from build123d import *

# Parameters (mm, degrees)
SKETCH1_W           = 40
SKETCH1_H           = 8
SKETCH1_W_2         = 4
BOSS_EXTRUDE1_DEPTH = 7.5
BOSS_EXTRUDE2_START = 2.75
SKETCH1_5_W         = 40
SKETCH1_5_H         = 8
SKETCH1_5_H_2       = 2
SKETCH1_5_W_2       = 4
BOSS_EXTRUDE2_DEPTH = 4.75
SKETCH1_7_R         = 1.65
BOSS_EXTRUDE3_DEPTH = 2.3
CUT_EXTRUDE3_START  = 2.3
SKETCH3_R           = 4.5
CUT_EXTRUDE3_DEPTH  = 47.651506616


with BuildPart() as part:
    # Sketch1 → Boss-Extrude1 (new body)
    with BuildSketch(Plane(origin=(0, 0, 0), x_dir=(0, 0, -1), z_dir=(1, 0, 0))):
        with Locations((20, 0)):
            Rectangle(SKETCH1_W, SKETCH1_H)
        with Locations((38, 0)):
            Rectangle(SKETCH1_W_2, SKETCH1_H)
    extrude(amount=BOSS_EXTRUDE1_DEPTH)

    # Sketch1<5> → Boss-Extrude2 (add)
    with BuildSketch(Plane(origin=(0, 0, 0), x_dir=(0, 0, -1), z_dir=(1, 0, 0)).offset(BOSS_EXTRUDE2_START)):
        with Locations((20, 0)):
            Rectangle(SKETCH1_5_W, SKETCH1_5_H)
        with Locations((20, 5)):
            Rectangle(SKETCH1_5_W, SKETCH1_5_H_2)
        with Locations((38, 0)):
            Rectangle(SKETCH1_5_W_2, SKETCH1_5_H)
        with Locations((38, 5)):
            Rectangle(SKETCH1_5_W_2, SKETCH1_5_H_2)
    extrude(amount=BOSS_EXTRUDE2_DEPTH)

    # Sketch1<7> → Boss-Extrude3 (add)
    with BuildSketch(Plane(origin=(0, 0, 0), x_dir=(0, 0, -1), z_dir=(1, 0, 0))):
        with BuildLine():
            Line((44, 4), (40, 4))
            Line((40, 4), (40, -4))
            Line((40, -4), (44, -4))
            ThreePointArc((44, -4), (48, 0), (44, 4))
        make_face()
        with Locations((44, 0)):
            Circle(SKETCH1_7_R, mode=Mode.SUBTRACT)
    extrude(amount=BOSS_EXTRUDE3_DEPTH)

    # Sketch3 → Cut-Extrude3 (cut, through all)
    with BuildSketch(Plane(origin=(0, 0, 0), x_dir=(0, 0, -1), z_dir=(1, 0, 0)).offset(CUT_EXTRUDE3_START)):
        with Locations((44, 0)):
            Circle(SKETCH3_R)
    extrude(amount=CUT_EXTRUDE3_DEPTH, mode=Mode.SUBTRACT)

    # Mirror1: part across plane


with BuildPart() as part_1:
    add(part.part)
    add(part.part.mirror(Plane(origin=(0, 0, 0), x_dir=(0, 0, 1), z_dir=(1, 0, 0))))

    # Mirror2: part across plane


with BuildPart() as part_2:
    add(part_1.part)
    add(part_1.part.mirror(Plane.XY))


solid = part_2.part
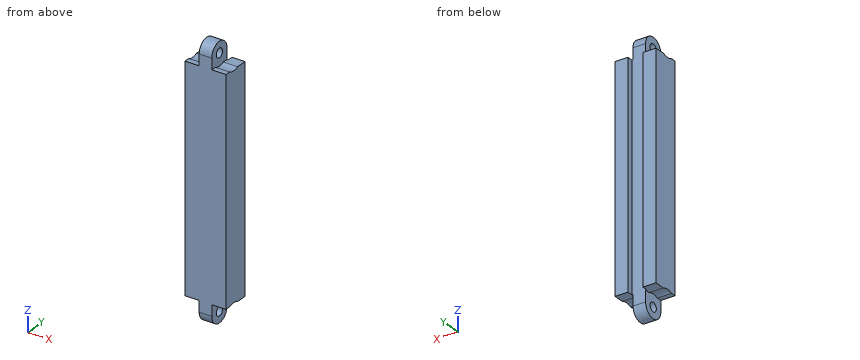
Read the model definition and answer for the solid it produces. Units are mm, in the model's axes. Give positions to 0.01 mm unless a question says otherwise; leave off trailing zeros. Write each loop counter-clockwise with the first axis right and the second up, starting at its lowest first coordinate (ties: lowest second). Pieces come first, ordered by that corner, then holes. Notation, with made-up numbers: (59.25, 2) - (72.25, 2) arc R30 ccw to (72.25, 41) - close; hole circle Ø4 at (87.25, -29). An arc over 180 degrees is marked (long way). Answer in a Markdown table with one row per item. Add a question column.
Item 1: Section A-A, the plane y = 0 is taken. Write down the section's boundary in (x, z).
Item 2: Flat-ended cylindrical pins translate along their axes: P1, Ø4.5, axis at x = 5.5, y = 5, coming from the +Z side; P2, Ø5, axis at x = 3.5, y = 2.5, coming from the +Z side; P3, Ø2, axis at x = -1, z = 3, coming from the +Y side. Find the tip coordinate at first contact, or state that the pin passes through.
Item 3: Section D-D, the plane x = 5.75 is taken. Write down the section's boundary in (y, z), and give its area (3 significant figures).
Item 4: Find the intervals of material crossed by L1, parallel to X at y = 4.25, z = 33; L2, parallel to Y at x = 0.8, z = -44; L3, parallel to Y at x = -1.75, z = 24.5, in increasing order.
Item 5: Section C-C, the plane x = 1.25 is taken. Write down the section's boundary in (y, z).
Item 6: Section B-B, the plane z = 7 is taken. Write down the section's boundary in (x, y).
Recorded:
| question | item | result |
|---|---|---|
| 1 | outline | (-7.5, -39.5) - (-2.3, -39.5) - (-2.3, -42.35) - (2.3, -42.35) - (2.3, -39.5) - (7.5, -39.5) - (7.5, 39.5) - (2.3, 39.5) - (2.3, 42.35) - (-2.3, 42.35) - (-2.3, 39.5) - (-7.5, 39.5) - close; (-2.3, -48) - (2.3, -48) - (2.3, -45.65) - (-2.3, -45.65) - close; (-2.3, 45.65) - (2.3, 45.65) - (2.3, 48) - (-2.3, 48) - close |
| 2 | P1 | stops at z = 40 |
| 2 | P2 | stops at z = 47.99 |
| 2 | P3 | stops at y = 4 |
| 3 | outline | (-4, -40) - (-2.06, -40) arc R4.5 cw to (2.06, -40) - (6, -40) - (6, 40) - (2.06, 40) arc R4.5 cw to (-2.06, 40) - (-4, 40) - close |
| 3 | area | 797 mm2 |
| 4 | L1 | x = -7.5 to -2.75, 2.75 to 7.5 |
| 4 | L2 | y = -4 to -1.65, 1.65 to 4 |
| 4 | L3 | y = -4 to 4 |
| 5 | outline | (-4, -44) arc R4 ccw to (4, -44) - (4, 44) arc R4 ccw to (-4, 44) - close; hole circle Ø3.3 at (0, -44); hole circle Ø3.3 at (0, 44) |
| 6 | outline | (-7.5, -4) - (7.5, -4) - (7.5, 6) - (2.75, 6) - (2.75, 4) - (-2.75, 4) - (-2.75, 6) - (-7.5, 6) - close |
